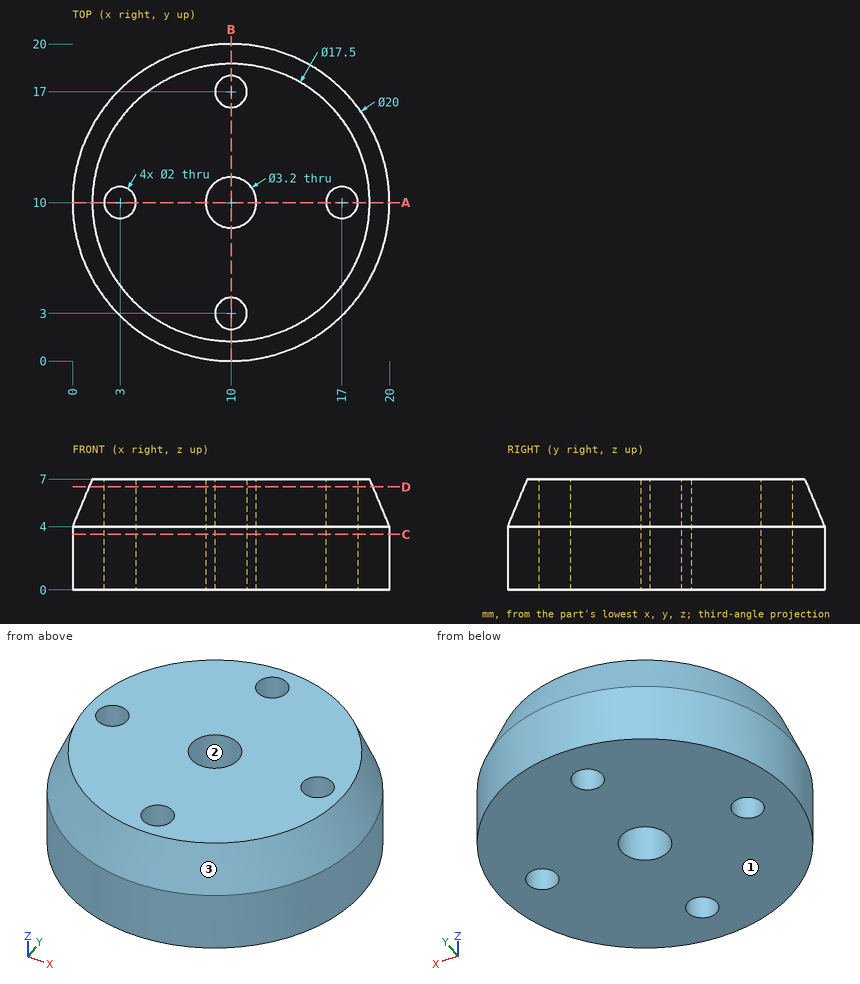
Job drawing, mm, ordinate dimensions from the low corner. One solid piece. Give positions to 0.01 mm unless a question says otherwise; leave off trailing zeros. Loops run counter-clockwise (first coordinate to the right, second up) from the corner with the lowest first, then second, coordinate; pieces in that order, holes last. Notation, with made-up numbers: M 85,35.5 L 96,35.5 A16 ccw 96,59.5 Z; hole C 24,17 d2. An arc over 180 degrees is marked long. Return JSON: item names as keys, results as strings.
1) Flat gauge pins, fed straight in: pin 1 Ø5 at (x, y) = (12, 3) entering from -Z; pin 2 Ø2 at (y, z) = (12.5, 4) entering from -X; pin 3 Ø2 at (y, z) = (11.5, 2.5) entering from -X; pin 4 Ø1 at (x, z) = (11.5, 5) entering from -Y. Where does each tip first touch, or does it go through?
Calculated:
{"pin 1": "stops at z = 0", "pin 2": "stops at x = 0.11", "pin 3": "stops at x = 0.01", "pin 4": "stops at y = 0.31"}
2) Pull direction Y, two halves, no side cores. Call the marked faces 1, 2 and 3: released by +Y, released by -Y, zero draft, split by the parting line, or undercut.
Calculated:
{"face 1": "zero draft", "face 2": "undercut", "face 3": "split by the parting line"}
3) Saw through at A-A, the plane y = 10. List the corners of the cut face in (x, z).
Calculated:
{"outline": "M 0,0 L 2,0 L 2,7 L 1.25,7 L 0,4 Z; M 4,0 L 8.4,0 L 8.4,7 L 4,7 Z; M 11.6,0 L 16,0 L 16,7 L 11.6,7 Z; M 18,0 L 20,0 L 20,4 L 18.75,7 L 18,7 Z"}
4) Saw through at C-C, the plane z = 3.5. List the corners of the cut face in (x, y), then the cut area to 3 significant figures.
Calculated:
{"outline": "C 10,10 d20; hole C 3,10 d2; hole C 10,10 d3.2; hole C 10,3 d2; hole C 10,17 d2; hole C 17,10 d2", "area": "294 mm2"}
5) Saw through at D-D, the plane z = 6.5. List the corners of the cut face in (x, y), then the cut area to 3 significant figures.
Calculated:
{"outline": "C 10,10 d17.92; hole C 3,10 d2; hole C 10,10 d3.2; hole C 10,3 d2; hole C 10,17 d2; hole C 17,10 d2", "area": "232 mm2"}
6) Drill centre lines: line 1 (Y direction, x = 10, z = 4.5); line 2 (Y direction, x = 10, z = 5.5) (3 decimals); line 3 (Y direction, x = 17, z = 3.75). Where is each one in solid material? Low to high.
Calculated:
{"line 1": "y = 0.21 to 2, 4 to 8.4, 11.6 to 16, 18 to 19.79", "line 2": "y = 0.625 to 2, 4 to 8.4, 11.6 to 16, 18 to 19.375", "line 3": "y = 2.86 to 9, 11 to 17.14"}
